Geometry: final body of the model. Coordinates: model frame, mm. A direction names the side the tool comes from. Round coordinates to 2 decimals unless told otherwise and drop trailing zeros. Loops run counter-clockwise (first coordinate to the right, second up) from the corner with the lowest first, then second, coordinate; pieces in that order, holes last. Notation, with made-up numbers: (70, -18) - (83, -18) arc R17 ccw to (83, 4) - close; hole circle Ø7 at (-36.5, 40.5). An arc over 180 degrees is marked (long way). Return JSON: item names as keys, results as strings. Group by question number.
1. Material intervals for probe 1 along Y at (x, z) = (12.25, 18.25); probe 2 along Y at (x, z) = (12.25, 14.25); probe 3 along Z at (x, y) = (6, 21), sorted ascending.
2. Section C-C on z = 23.5. Return loops of the section in (x, y), and give its area (3 significant figures).
3. Section A-A on z = 12.7. Return loops of the section in (x, y).
4. Section B-B on y = 27. Return loops of the section in (x, z), and give its area (3 significant figures).
5. Draft query along X for faces 1 (the face through (-1.46, 34.37, 15.74)), 2 (the face through (12, 23, 8.117)), 3 (the face through (6.535, 22.678, 19.542)), 4 (the face through (-1.4, 22.68, 19.61)). Return one class per face: +X half, -X half, draft (parallel to the pull), parting line (faces both ways), or undercut.
6. Section D-D on y = 31.75. Return loops of the section in (x, z).
7. First-contact query: pin 1 Ø6 at (y, z) = (22, 22) entering from +X; pin 2 Ø2 at (x, y) = (12.5, 24) entering from +Z; pin 3 Ø5 at (x, z) = (4.5, 10.5) entering from -Y. Flat tips, straight axial feed; report the tip coordinate or a pass-through.
8. Set-up query: faces 5 (the face through (-6, 20.173, 13)), 6 (the face through (-5.427, 23, 13)), 7 (the face through (2, 27.753, 23)), 8 (the face through (6.42, 22.68, 5.79)). Return all of +Z, -Z, +X, -X, +Y, -Y with unobstructed straight access to the full face (end or side cutting, diameter ignored); none if empty.
from build123d import *

# Parameters (mm, degrees)
BOSS_EXTRUDE1_DEPTH = 25.4
BOSS_EXTRUDE3_DEPTH = 5.08
SKETCH4_W           = 37.4
SKETCH4_H           = 25.4
CUT_EXTRUDE1_DEPTH  = 25.4
SKETCH5_R           = 12.7
BOSS_EXTRUDE4_DEPTH = 2.5
SKETCH6_R           = 5
BOSS_EXTRUDE5_DEPTH = 8.272
FILLET1_R           = 5


with BuildPart() as part:
    # Sketch1 → Boss-Extrude1 (new body)
    with BuildSketch(Plane.XY):
        Polygon((-10.189534884, 0), (-10.189534884, 9), (15.210465116, 9), (15.210465116, 0), (21.210465116, 0), (21.210465116, 20.17346), (-16.189534884, 20.17346), (-16.189534884, 0), align=None)
    extrude(amount=BOSS_EXTRUDE1_DEPTH)

    # Sketch3 → Boss-Extrude3 (add)
    with BuildSketch(Plane(origin=(0, 20.17346, 0), x_dir=(1, 0, 0), z_dir=(0, 1, 0))):
        with BuildLine():
            Line((14.354818113, -17.282717762), (10.447965116, -17.282717762))
            Line((10.447965116, -17.282717762), (2.510465116, -21.865435523))
            Line((2.510465116, -21.865435523), (-5.427034884, -17.282717762))
            Line((-5.427034884, -17.282717762), (-5.427034884, -8.117282238))
            Line((-5.427034884, -8.117282238), (2.510465116, -3.534564477))
            Line((2.510465116, -3.534564477), (10.447965116, -8.117282238))
            Line((10.447965116, -8.117282238), (14.354818113, -8.117282238))
            ThreePointArc((14.354818113, -8.117282238), (-10.189534884, -12.7), (14.354818113, -17.282717762))
        make_face()
    extrude(amount=BOSS_EXTRUDE3_DEPTH)

    # Sketch4 → Cut-Extrude1 (cut)
    with BuildSketch(Plane(origin=(0, 20.17346, 0), x_dir=(1, 0, 0), z_dir=(0, 1, 0))):
        with Locations((2.510465116, -12.7)):
            Rectangle(SKETCH4_W, SKETCH4_H)
    extrude(amount=-CUT_EXTRUDE1_DEPTH, mode=Mode.SUBTRACT)

    # Sketch5 → Boss-Extrude4 (add)
    with BuildSketch(Plane(origin=(0, 25.25346, 0), x_dir=(1, 0, 0), z_dir=(0, 1, 0))):
        with Locations((2.510465116, -12.7)):
            Circle(SKETCH5_R)
    extrude(amount=BOSS_EXTRUDE4_DEPTH)

    # Sketch6 → Boss-Extrude5 (add)
    with BuildSketch(Plane(origin=(0, 27.75346, 0), x_dir=(1, 0, 0), z_dir=(0, 1, 0))):
        with Locations((2.510465116, -12.7)):
            Circle(SKETCH6_R)
    extrude(amount=BOSS_EXTRUDE5_DEPTH)

    # Fillet1
    fillet1_edges = [part.edges().sort_by_distance(p)[0] for p in [
        (-2.489534884, 27.75346, 12.7),
    ]]
    fillet(fillet1_edges, radius=FILLET1_R)


solid = part.part
Taken from the geometry:
{
 "1": {"probe 1": "20.17 to 27.75", "probe 2": "25.25 to 27.76", "probe 3": "0.49 to 5.55, 19.85 to 24.91"},
 "2": {"outline": "(-4.17, 20.17) - (9.19, 20.17) - (9.19, 27.75) - (-4.17, 27.75) - close", "area": "101 mm2"},
 "3": {"outline": "(-10.19, 20.17) - (-5.43, 20.17) - (-5.43, 25.25) - (15.21, 25.25) - (15.21, 27.75) - (12.51, 27.75) arc R5 cw to (7.51, 32.75) - (7.51, 36.03) - (-2.49, 36.03) - (-2.49, 32.75) arc R5 cw to (-7.49, 27.75) - (-10.19, 27.75) - close"},
 "4": {"outline": "circle Ø25.4 at (2.51, 12.7)", "area": "507 mm2"},
 "5": {"face 1": "parting line", "face 2": "draft", "face 3": "undercut", "face 4": "undercut"},
 "6": {"outline": "circle Ø10.2 at (2.51, 12.7)"},
 "7": {"pin 1": "x = 13.54", "pin 2": "z = 21.67", "pin 3": "y = 25.25"},
 "8": {"face 5": "+Z, -Z, +X, -X, -Y", "face 6": "+X, -Y", "face 7": "+Y", "face 8": "-Y"}
}
